The drawing under review shows one solid part. Ordinate dimensions are in mm from its lowest x, y, z. A direction names the side the tool comes from. Coordinates: 2 decimals unless noted, no trailing zeros. Return JSON: item names as keys, results as strings.
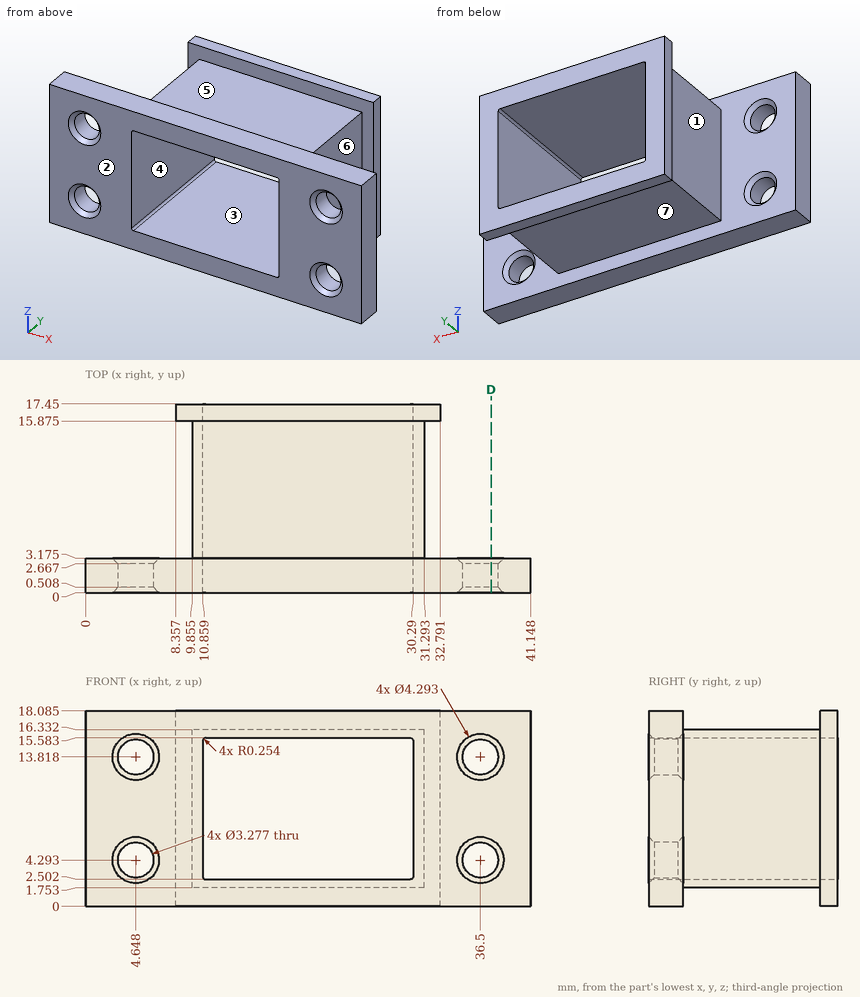
1. Add section D-D on x = 37.5. State how many separate pieces and enclosed holes the cut face has, plus the area to 3 significant figures.
Check values:
{"separate pieces": "3", "enclosed holes": "0", "area": "39.7 mm²"}
2. To check wall thickness, follow line 1 (Z direction, x = 29.5, y = 9); line 2 (X direction, y = 12.25, z = 7) (1 decimal); line 3 (X direction, y = 16.5, z = 9). State the ranges of each line that lie inside material, in increasing order.
Check values:
{"line 1": "1.75 to 2.5, 15.58 to 16.33", "line 2": "9.9 to 10.9, 30.3 to 31.3", "line 3": "8.36 to 10.86, 30.29 to 32.79"}
3. Insertion check: pin 1 Ø8.5 at (x, y) = (24, 11) entering from -Z; pin 2 Ø3 at (y, z) = (15.5, 13) entering from -X; pin 3 Ø0.5 at (y, z) = (17, 12) entering from +X. Each pin has a flat end and moves straight along its axis. Give the tip position at first contact, or say it passes through.
Check values:
{"pin 1": "z = 1.75", "pin 2": "x = 8.36", "pin 3": "x = 32.79"}
4. Machinability: for the marked faces 4, 5, 6 and 7, which of the approach directions +Z, -Z, +X, -X, +Y, -Y give a long, thin tool a straight path to every point of the face, cutting with its end or side? Answer none if there is none.
Check values:
{"face 4": "+Y, -Y", "face 5": "+Z, +X, -X", "face 6": "+Z, -Z, +X", "face 7": "-Z, +X, -X"}
5. The part is to be moulded in two halves that separate along X. For the marked faces 1, 2 and 3, say which applies: released by +X, released by -X, zero draft, split by the parting line, or undercut.
Check values:
{"face 1": "released by -X", "face 2": "zero draft", "face 3": "undercut"}
